The model under review builds one solid part; all positions refer to its coordinate system, in mm. A direction names the side the tool comes from. Coordinates: 2 decimals unless noted, no trailing zeros. Write each loop counter-clockwise with the first axis right and the second up, starting at its lowest first coordinate (ties: lowest second). Pieces come first, ordered by that corner, then holes. Notation, with made-up numbers: (55, 12) -> (98, 12) arc R28 cw to (98, 51) -> close; hole circle Ø7 at (-4, 5.5). An arc over 180 degrees is marked (long way). Write each question's results on one line, items separated by ' | '.
```python
from build123d import *

# Parameters (mm, degrees)
SKETCH1_R               = 18
BOSS_EXTRUDE1_DEPTH     = 30
FILLET1_R               = 3
SKETCH2_W               = 10
SKETCH2_H               = 10
CUT_EXTRUDE1_DEPTH      = 25
SKETCH3_R               = 1.6
CUT_EXTRUDE2_DEPTH      = 24
CUT_EXTRUDE2_DEPTH_BACK = 14.0000001
CUT_EXTRUDE3_START      = -9
SKETCH4_R               = 3.5
CUT_EXTRUDE3_DEPTH      = 20
CUT_EXTRUDE4_START      = -8
CUT_EXTRUDE4_DEPTH      = 16


with BuildPart() as part:
    # Sketch1 → Boss-Extrude1 (new body)
    with BuildSketch(Plane(origin=(0, 0, 0), x_dir=(1, 0, 0), z_dir=(0, 1, 0))):
        Circle(SKETCH1_R)
    extrude(amount=BOSS_EXTRUDE1_DEPTH)

    # Fillet1
    fillet1_edges = [part.edges().sort_by_distance(p)[0] for p in [
        (-18, 30, 0),
    ]]
    fillet(fillet1_edges, radius=FILLET1_R)

    # Sketch2 → Cut-Extrude1 (cut)
    with BuildSketch(Plane.XZ):
        Rectangle(SKETCH2_W, SKETCH2_H)
    extrude(amount=-CUT_EXTRUDE1_DEPTH, mode=Mode.SUBTRACT)

    # Sketch3 → Cut-Extrude2 (cut, two sides)
    with BuildSketch(Plane.ZY.offset(-5)) as cut_extrude2_sk:
        with Locations((0, 6)):
            Circle(SKETCH3_R)
    extrude(amount=CUT_EXTRUDE2_DEPTH, mode=Mode.SUBTRACT)
    extrude(cut_extrude2_sk.sketch, amount=-CUT_EXTRUDE2_DEPTH_BACK, mode=Mode.SUBTRACT)

    # Sketch4 → Cut-Extrude3 (cut)
    with BuildSketch(Plane.ZY.offset(-5).offset(CUT_EXTRUDE3_START)):
        with Locations((0, 6)):
            Circle(SKETCH4_R)
    extrude(amount=-CUT_EXTRUDE3_DEPTH, mode=Mode.SUBTRACT)

    # Sketch5 → Cut-Extrude4 (cut)
    with BuildSketch(Plane(origin=(-5, 0, 0), x_dir=(0, 0, -1), z_dir=(1, 0, 0)).offset(CUT_EXTRUDE4_START)):
        Polygon((-2.814582562, 7.625), (-2.814582562, 4.375), (0, 2.75), (2.814582562, 4.375), (2.814582562, 7.625), (0, 9.25), align=None)
    extrude(amount=-CUT_EXTRUDE4_DEPTH, mode=Mode.SUBTRACT)


solid = part.part
```
Q1. Clearance check with flat-ended pins moving along their axes: P1, Ø2.5, axis at x = -14.5, y = 5.5, coming from the +Z side; P2, Ø1.5, axis at x = -14, y = 25.5, coming from the -Z side; P3, Ø3, axis at y = 6, z = 0, coming from the +X side; P4, Ø1, axis at x = -14.5, y = 6.5, coming from the -Z side. State where each tip first meets the part, or that it passes through.
Solution:
P1: z = 12.18 | P2: z = -12.18 | P3: through | P4: z = -11.31
Q2. Draft analysis for pull direction Y (two halves, no side actions). For faces 4 (the flat face through (14, 4, 1)), 5 (the flat face through (0, 12, -5)), 6 (the flat face through (0, 0, 8)), state which applies: pulls with the +Y half, pulls with the -Y half, needs draft (parallel to the pull), parting line crosses it, or undercut.
Solution:
face 4: undercut | face 5: needs draft | face 6: pulls with the -Y half
Q3. Add section A-A (x = 0). Write out the cut boundary in (y, z).
Solution:
outline: (0, -18) -> (27, -18) arc R3 ccw to (30, -15) -> (30, 15) arc R3 ccw to (27, 18) -> (0, 18) -> (0, 5) -> (25, 5) -> (25, -5) -> (0, -5) -> close
Q4. Machinability: for faces 1 (the cylindrical face through (15.972, 6.154, -3.497)), 2 (the flat face through (-15.465, 3.551, -1.388)), 3 (the flat face through (0, 25, 0)), which of the approach directions +Z, -Z, +X, -X, +Y, -Y give a long, thin tool a straight path to every point of the face, cutting with its end or side? Answer none if there is none.
Solution:
face 1: +X | face 2: -X | face 3: -Y
Q5. Add section B-B (y = 6). Write out the cut boundary in (x, z), plus the area to 3 significant figures.
Solution:
outline: (-17.78, -2.81) arc R18 ccw to (17.66, -3.5) -> (14, -3.5) -> (14, -1.6) -> (5, -1.6) -> (5, -5) -> (-5, -5) -> (-5, -1.6) -> (-13, -1.6) -> (-13, -2.81) -> close; (-17.78, 2.81) -> (-13, 2.81) -> (-13, 1.6) -> (-5, 1.6) -> (-5, 5) -> (5, 5) -> (5, 1.6) -> (14, 1.6) -> (14, 3.5) -> (17.66, 3.5) arc R18 ccw to start | area: 809 mm²
Q6. For line 1 (Y direction, x = -8, z = 0); line 2 (Z direction, x = -10, y = 6); line 3 (Y direction, x = -4, z = -3), list the stretches that pass through material, from the lowest coordinate up. Write a range as from..to.
Solution:
line 1: 0..4.4, 7.6..30 | line 2: -14.97..-1.6, 1.6..14.97 | line 3: 25..30
